from build123d import *

# Parameters (mm, degrees)
SZKIC1_W                    = 55
SZKIC1_H                    = 45
DODANIE_WYCI_GNI_CIE1_DEPTH = 2
ZAOKR_GLENIE1_R             = 10
ZAOKR_GLENIE2_R             = 10
SZKIC2_R                    = 3
WYTNIJ_WYCI_GNI_CIE2_DEPTH  = 2


with BuildPart() as part:
    # Szkic1 → Dodanie-wyciągnięcie1 (new body)
    with BuildSketch(Plane.XY):
        with Locations((0, 721.92245047)):
            Rectangle(SZKIC1_W, SZKIC1_H)
    extrude(amount=DODANIE_WYCI_GNI_CIE1_DEPTH)

    # Zaokrąglenie1
    zaokr_glenie1_edges = [part.edges().sort_by_distance(p)[0] for p in [
        (-27.5, 699.42245047, 1),
    ]]
    fillet(zaokr_glenie1_edges, radius=ZAOKR_GLENIE1_R)

    # Zaokrąglenie2
    zaokr_glenie2_edges = [part.edges().sort_by_distance(p)[0] for p in [
        (27.5, 699.42245047, 1),
    ]]
    fillet(zaokr_glenie2_edges, radius=ZAOKR_GLENIE2_R)

    # Szkic2 → Wytnij-wyciągnięcie2 (cut)
    with BuildSketch(Plane.XY.offset(2)):
        with Locations((0, 716.42245047)):
            Circle(SZKIC2_R)
    extrude(amount=-WYTNIJ_WYCI_GNI_CIE2_DEPTH, mode=Mode.SUBTRACT)


solid = part.part
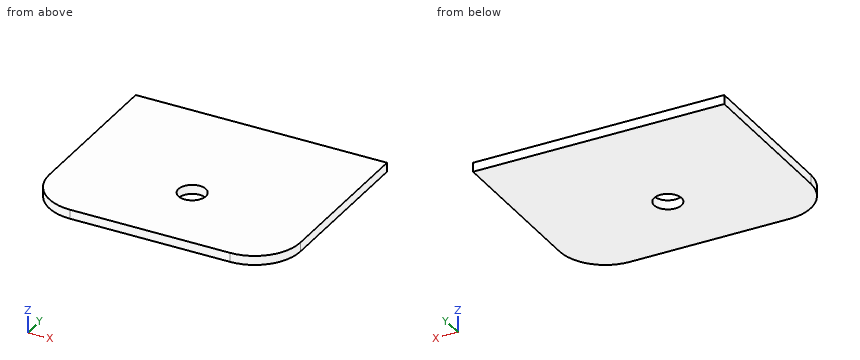
Check sheet for the modelled part. Datum: model origin and axes. Units: mm. Give positions to 0.01 mm unless a question says otherwise; leave off trailing zeros. Loops run counter-clockwise (first coordinate to the right, second up) from the corner with the lowest first, then second, coordinate; pieces in that order, holes last. Notation, with made-up numbers: M 12.25,-7.75 L 40.25,-7.75 A21 ccw 40.25,1.25 Z; hole C 72.25,-37 d9. An arc over 180 degrees is marked long. Return JSON: item names as keys, results as strings. Group by question number.
1. Cross-section at A-A on x = 0. Record the boundary of the cut face in (y, z), plus the area to 3 significant figures.
2. Cross-section at B-B on z = 1.2. Record the boundary of the cut face in (x, y).
3. Thickness scan on L1, parallel to Y at x = 0, z = 1.1; L2, parallel to Y at x = 1, z = 0.65; L3, parallel to X at y = 719, z = 0.7 (3 decimals). Record the ranges inside material, lowest first.
4. Go/stop test with a flat-tipped pin: pin 1 (5 mm diameter, centred on x = 0, y = 716.42, fed in from -Z). Record where the tip stops, or that it passes through.
5. Cross-section at C-C on y = 706. Record the boundary of the cut face in (x, z), plus the area to 3 significant figures.
Return value:
{
 "1": {"outline": "M 699.42,0 L 713.42,0 L 713.42,2 L 699.42,2 Z; M 719.42,0 L 744.42,0 L 744.42,2 L 719.42,2 Z", "area": "78.0 mm^2"},
 "2": {"outline": "M -27.5,709.42 A10 ccw -17.5,699.42 L 17.5,699.42 A10 ccw 27.5,709.42 L 27.5,744.42 L -27.5,744.42 Z; hole C 0,716.42 d6"},
 "3": {"L1": "699.42 to 713.42, 719.42 to 744.42", "L2": "699.42 to 713.59, 719.25 to 744.42", "L3": "-27.5 to -1.535, 1.535 to 27.5"},
 "4": {"pin 1": "through"},
 "5": {"outline": "M -26.9,0 L 26.9,0 L 26.9,2 L -26.9,2 Z", "area": "108 mm^2"}
}
